```python
from build123d import *
from build123d.topology import SkipClean

# Parameters (mm, degrees)
BOSS_EXTRUDE1_START     = 34.9504
BOSS_EXTRUDE1_DEPTH     = 34.9504
BOSS_EXTRUDE2_DEPTH     = 17.4752001
SKETCH5_R               = 12.1539
CUT_EXTRUDE1_DEPTH      = 34.9504
CUT_EXTRUDE2_REACH      = 66.019
CUT_EXTRUDE2_END_RADIUS = 12.1539
SKETCH6_R               = 12.1539


# Read off the part's stored shape, not the designer's step: Boss-Extrude2
with BuildPart() as part:
    # Sketch1 → Revolve1 (revolve)
    with BuildSketch(Plane.XY, mode=Mode.PRIVATE) as revolve1_sk:
        Polygon((-46.1772, -21.3741), (-17.4752, -21.3741), (-17.4752, -16.637), (-46.1772, -16.8275), align=None)
    revolve(revolve1_sk.sketch.rotate(Axis((-46.1772, 0, 0), (1, 0, 0)), 270), axis=Axis((-46.1772, 0, 0), (1, 0, 0)))


with BuildPart() as body_2:
    # Mirror1: mirrored copy
    add(part.part.mirror(Plane(origin=(0, 0, 0), x_dir=(0, 0, 1), z_dir=(1, 0, 0))))


with BuildPart() as body_3:
    # Sketch2 → Revolve2 (revolve)
    with BuildSketch(Plane.XY, mode=Mode.PRIVATE) as revolve2_sk:
        Polygon((16.8275, 46.1772), (16.637, 17.4752), (21.3741, 17.4752), (21.3741, 46.1772), align=None)
    revolve(revolve2_sk.sketch.rotate(Axis((0, 0, 0), (0, 1, 0)), 90), axis=Axis((0, 0, 0), (0, 1, 0)))


with BuildPart() as part_1:
    with SkipClean():  # the faces are left unmerged after this step: merging them gives an invalid solid
        add(part.part)

        add(body_2.part)  # Boss-Extrude1 merges body 2

        add(body_3.part)  # Boss-Extrude1 merges body 3
        # Sketch3 → Boss-Extrude1 (add)
        with BuildSketch(Plane(origin=(-17.4752, 0, 0), x_dir=(0, 0, -1), z_dir=(1, 0, 0)).offset(BOSS_EXTRUDE1_START)):
            with BuildLine():
                Line((12.307296038, 17.4752), (-12.307296038, 17.4752))
                ThreePointArc((-12.307296038, 17.4752), (0, -21.3741), (12.307296038, 17.4752))
            make_face()
        extrude(amount=-BOSS_EXTRUDE1_DEPTH)

    # Boss-Extrude2 outline → Boss-Extrude2 (add)
    with SkipClean():  # the faces are left unmerged after this step: merging them gives an invalid solid
        with BuildSketch(Plane.XZ.offset(-17.4752)):
            with BuildLine():
                ThreePointArc((-17.4752, -12.307296038), (0, -21.3741), (17.4752, -12.307296038))
                Line((17.4752, -12.307296038), (17.4752, 12.307296038))
                ThreePointArc((17.4752, 12.307296038), (0, 21.3741), (-17.4752, 12.307296038))
                Line((-17.4752, 12.307296038), (-17.4752, -12.307296038))
            make_face()
        extrude(amount=BOSS_EXTRUDE2_DEPTH)

    # Sketch5 → Cut-Extrude1 (cut)
    with SkipClean():  # the faces are left unmerged after this step: merging them gives an invalid solid
        with BuildSketch(Plane.ZY.offset(17.4752)):
            Circle(SKETCH5_R)
        extrude(amount=-CUT_EXTRUDE1_DEPTH, mode=Mode.SUBTRACT)

    # Cut-Extrude2: up to this cylinder (the profile starts outside it)
    with SkipClean():  # the faces are left unmerged after this step: merging them gives an invalid solid
        cut_extrude2_end = Plane(origin=(0, 0, 0), z_dir=(-1, 0, 0)) * Cylinder(CUT_EXTRUDE2_END_RADIUS, 157.3458, mode=Mode.PRIVATE)
        # Sketch6 → Cut-Extrude2 (cut, up to the surface)
        with BuildSketch(Plane(origin=(0, 17.4752, 0), x_dir=(1, 0, 0), z_dir=(0, 1, 0)), mode=Mode.PRIVATE) as cut_extrude2_sk1:
            with Locations(Location((0, 0, 0), (0, 0, 270))):
                Circle(SKETCH6_R)
        cut_extrude2_tool1 = extrude(cut_extrude2_sk1.sketch, amount=-CUT_EXTRUDE2_REACH, mode=Mode.PRIVATE) - cut_extrude2_end
        add(cut_extrude2_tool1.solids().sort_by_distance((0, 17.4752, 0))[0], mode=Mode.SUBTRACT)


solid = part_1.part
```
Check sheet for the modelled part. Datum: model origin and axes. Units: mm. A direction names the side the tool comes from. Coordinates: 2 decimals unless noted, no trailing zeros. Loops run counter-clockwise (first coordinate to the right, second up) from the corner with the lowest first, then second, coordinate; pieces in that order, holes last.
1) Access from +Z, -Z, +X, -X, +Y, -Y to the whole of each face (thin tool, end or side, straight path). Record for faces 1 (the face through (-32.03, -5.03, 15.96)), 2 (the face through (32.03, -5.03, 15.96)), 3 (the face through (-0.245, -11.865, -2.635)), 4 (the face through (-9.8, 17.475, -7.5)).
2) Sectioned sample at B-B (y = 26). Record the boundary of the cut face in (x, z).
3) Release check for a two-part mould opening along Z. For faces 5 (the face through (46.177, 16, -6)), 6 (the face through (0.534, 12.743, -12.142)) record: released by +Z, released by -Z, zero draft, split by the parting line, or undercut.
4) Material ranges on probe 1 along Z at (x, y) = (9.5, 0); probe 2 along X at (y, z) = (13, 0); probe 3 along Y at (x, z) = (-9, 0), recorded low to high.
5) Sectioned sample at C-C (x = -33). Record the boundary of the cut face in (y, z), and give its area (3 significant figures).
6) Gauge pin test, flat ends, axial feed: pin 1 (6 mm diameter, centred on x = 10, y = 7, fed in from -Z); pin 2 (22 mm diameter, centred on y = 0, z = 0, fed in from +X); pin 3 (19.5 mm diameter, centred on x = 0, z = 0, fed in from -Y); pin 4 (8.5 mm diameter, centred on y = 12, z = 2.5, fed in from -X). Record the tip position at first contact, or that the pin passes through.
7) Sectioned sample at A-A (z = 0). Count the separate pieces of the cut face and the enclosed holes in it, and give its area (3 significant figures).
Check sheet entries:
1. face 1: -X
1. face 2: +X
1. face 3: +X, -X
1. face 4: +Y
2. outline: circle Ø42.75 at (0, 0); hole circle Ø33.39 at (0, 0)
3. face 5: zero draft
3. face 6: undercut
4. probe 1: z = -21.37 to -12.15, 12.15 to 21.37
4. probe 2: x = -17.48 to -12.15, 12.15 to 17.48
4. probe 3: y = -21.37 to -12.15
5. outline: circle Ø42.75 at (0, 0); hole circle Ø33.48 at (0, 0)
5. area: 555 mm2
6. pin 1: stops at z = -21
6. pin 2: passes through
6. pin 3: stops at y = -21.37
6. pin 4: stops at x = -17.48
7. separate pieces: 3
7. enclosed holes: 0
7. area: 1,150 mm2
